```python
from build123d import *

# Parameters (mm, degrees)
SKETCH1_W           = 27.5
SKETCH1_H           = 27.5
BOSS_EXTRUDE3_DEPTH = 15
CUT_EXTRUDE1_DEPTH  = 10
SKETCH4_W           = 17.8
SKETCH4_H           = 17.8
BOSS_EXTRUDE4_DEPTH = 10
BOSS_EXTRUDE5_DEPTH = 15


with BuildPart() as part:
    # Sketch1 → Boss-Extrude3 (new body)
    with BuildSketch(Plane(origin=(0, 0, 0), x_dir=(1, 0, 0), z_dir=(0, 1, 0))):
        Rectangle(SKETCH1_W, SKETCH1_H)
    extrude(amount=BOSS_EXTRUDE3_DEPTH)

    # Sketch3 → Cut-Extrude1 (cut)
    with BuildSketch(Plane(origin=(0, 15, 0), x_dir=(1, 0, 0), z_dir=(0, 1, 0))):
        Polygon((-13.75, -13.75), (-8.55, -13.75), (-8.55, 8.55), (13.75, 8.55), (13.75, 13.75), (-13.75, 13.75), align=None)
    extrude(amount=-CUT_EXTRUDE1_DEPTH, mode=Mode.SUBTRACT)

    # Sketch4 → Boss-Extrude4 (add)
    with BuildSketch(Plane(origin=(0, 15, 0), x_dir=(1, 0, 0), z_dir=(0, 1, 0))):
        with Locations((2.6, -2.6)):
            Rectangle(SKETCH4_W, SKETCH4_H)
    extrude(amount=BOSS_EXTRUDE4_DEPTH)

    # Sketch6 → Boss-Extrude5 (add)
    with BuildSketch(Plane.XZ):
        Polygon((-11.35, -11.35), (-11.35, 13.75), (-13.75, 13.75), (-13.75, -13.75), (13.75, -13.75), (13.75, -11.35), align=None)
    extrude(amount=BOSS_EXTRUDE5_DEPTH)


solid = part.part
```
Could you check a few things on this model? Use its own coordinates, in mm. A direction names the side the tool comes from. Round coordinates to 2 decimals unless told otherwise and drop trailing zeros. Loops run counter-clockwise (first coordinate to the right, second up) from the corner with the lowest first, then second, coordinate; pieces in that order, holes last. Notation, with made-up numbers: M 67.5,-2 L 104.5,-2 A17 cw 104.5,12 Z; hole C 45.25,19 d9. An arc over 180 degrees is marked long. Put each result on its own line as item: value.
Q1. On a 3-axis mill with a long thin cutter (end or side, diameter ignored), from which of +Z, -Z, +X, -X, +Y, -Y can I reach the whole of each face in a straight line? I mean faces 1 (the face through (2, 10, -8.55)), 2 (the face through (2, 20, 11.5)), 3 (the face through (-11.35, -7, 1)), 4 (the face through (-8.55, 10, 3)), 5 (the face through (11.5, 20, 3)). Say none if no direction works.
Check result:
face 1: -Z, +X, -X, +Y
face 2: +Z, +X, -X, +Y
face 3: +Z, +X, -Y
face 4: +Z, -Z, -X, +Y
face 5: +Z, -Z, +X, +Y
Q2. Imagine slicing it at D-D (z = -10.5). Write out the boundary of the cut face in (x, y).
Check result:
outline: M -13.75,-15 L -11.35,-15 L -11.35,0 L 13.75,0 L 13.75,5 L -13.75,5 Z
Q3. I need wall thicknesses on probe 1 along X at (y, z) = (-11, -2.5); probe 2 along Z at (x, y) = (1.25, 12); probe 3 along Y at (x, z) = (-9.75, 9). Which ranges of each line are inside material? Lowest first, please.
Check result:
probe 1: -13.75 to -11.35
probe 2: -8.55 to 13.75
probe 3: 0 to 5
Q4. For pin 1 (12 mm diameter, centred on x = -1.5, y = -4, fed in from +Z); pin 2 (7.5 mm diameter, centred on x = 3.5, y = -6, fed in from +Z); pin 3 (5 mm diameter, centred on y = 22, z = -0.5, fed in from -X); pin 4 (5 mm diameter, centred on x = 3, y = 10.5, fed in from -Z), each with a flat end and sliding along its axis, tell me the tip position at first contact or that it passes through.
Check result:
pin 1: z = 13.75
pin 2: z = -11.35
pin 3: x = -6.3
pin 4: z = -8.55
Q5. Imagine slicing it at B-B (x = 0). Write out the boundary of the cut face in (y, z).
Check result:
outline: M -15,-13.75 L 5,-13.75 L 5,-8.55 L 15,-8.55 L 15,-6.3 L 25,-6.3 L 25,11.5 L 15,11.5 L 15,13.75 L 0,13.75 L 0,-11.35 L -15,-11.35 Z
Q6. Imagine slicing it at C-C (y = -12). Write out the boundary of the cut face in (x, z).
Check result:
outline: M -13.75,-13.75 L 13.75,-13.75 L 13.75,-11.35 L -11.35,-11.35 L -11.35,13.75 L -13.75,13.75 Z
Q7. Imagine slicing it at A-A (z = -7). Write out the boundary of the cut face in (x, y), then the cut area to 4 significant figures.
Check result:
outline: M -13.75,-15 L -11.35,-15 L -11.35,0 L 13.75,0 L 13.75,15 L -8.55,15 L -8.55,5 L -13.75,5 Z
area: 396.5 mm2
